```python
from build123d import *

# Parameters (mm, degrees)
F0_W     = 60
F0_H     = 100
F0_R     = 17.5
F1_DEPTH = 20
F2_W     = 100
F2_H     = 20
F2_R     = 5
F3_DEPTH = 100
F4_R     = 4.99999


# Not quite as in the source:
# - a fillet or chamfer is up to 0.001 mm smaller than in the source, because OpenCascade refuses the exact size


with BuildPart() as f1:
    # F0 (on Top) → F1 (new body)
    with BuildSketch(Plane.XY):
        Rectangle(F0_W, F0_H)
        Circle(F0_R, mode=Mode.SUBTRACT)
    extrude(amount=F1_DEPTH)

    # F2 (on face) → F3 (intersect)
    with BuildSketch(Plane.YZ.offset(30)):
        with Locations((0, 10)):
            Rectangle(F2_W, F2_H)
        with Locations((-35, 10)):
            Circle(F2_R, mode=Mode.SUBTRACT)
        with Locations((35, 10)):
            Circle(F2_R, mode=Mode.SUBTRACT)
    extrude(amount=-F3_DEPTH, mode=Mode.INTERSECT)

    # F4 (radius 5 in the source; OpenCascade refuses exactly that, so slightly less here)
    f4_edges = [f1.edges().sort_by_distance(p)[0] for p in [
        (30, 0, 20),
        (0, -50, 20),
        (-30, 0, 20),
        (0, 50, 20),
    ]]
    fillet(f4_edges, radius=F4_R)


solid = f1.part
```
For this review, take the finished solid that the model builds, in its own axes (mm). Round coordinates to 2 decimals unless told otherwise and drop trailing zeros. Write each loop counter-clockwise with the first axis right and the second up, starting at its lowest first coordinate (ties: lowest second). Pieces come first, ordered by that corner, then holes. Notation, with made-up numbers: (-15.75, 7.25) - (23.25, 7.25) arc R27 ccw to (23.25, 27.25) - close; hole circle Ø4 at (11.5, 39.25). An arc over 180 degrees is marked (long way). Write each question's results on one line, items separated by ' | '.
Item 1: For pin 1 (9 mm diameter, centred on y = 35, z = 10, fed in from +X), flat-tipped, find the tip position at first contact; note if it passes through.
Calculated:
pin 1: passes through
Item 2: Take a section at C-C on y = -31. State the section outline as (x, z) points, then the cut area to 3 significant figures.
Calculated:
outline: (-30, 0) - (30, 0) - (30, 7) - (-30, 7) - close; (-30, 13) - (30, 13) - (30, 15) arc R5 ccw to (25, 20) - (-25, 20) arc R5 ccw to (-30, 15) - close | area: 829 mm^2
Item 3: To check wall thickness, follow line 1 along Z through (x, y) = (7, 35); line 2 along Y through (x, z) = (27, 9.5); line 3 along Y through (x, z) = (0, 4.5). State the ranges of each line that lie inside material, in increasing order. Write a range as from..to.
Calculated:
line 1: z = 0..5, 15..20 | line 2: y = -50..-39.97, -30.03..30.03, 39.97..50 | line 3: y = -50..-17.5, 17.5..50
Item 4: Take a section at B-B on z = 10. State the section outline as (x, y) points.
Calculated:
outline: (-30, -50) - (30, -50) - (30, -40) - (-30, -40) - close; (-30, -30) - (30, -30) - (30, 30) - (-30, 30) - close; (-30, 40) - (30, 40) - (30, 50) - (-30, 50) - close; hole circle Ø35 at (0, 0)
Item 5: Take a section at D-D on x = -24. State the section outline as (y, z) points.
Calculated:
outline: (-50, 0) - (50, 0) - (50, 15) arc R5 ccw to (45, 20) - (-45, 20) arc R5 ccw to (-50, 15) - close; hole circle Ø10 at (-35, 10); hole circle Ø10 at (35, 10)
Item 6: Take a section at A-A on x = 0. State the section outline as (y, z) points, then the cut area to 3 significant figures.
Calculated:
outline: (-50, 0) - (-17.5, 0) - (-17.5, 20) - (-45, 20) arc R5 ccw to (-50, 15) - close; (17.5, 0) - (50, 0) - (50, 15) arc R5 ccw to (45, 20) - (17.5, 20) - close; hole circle Ø10 at (-35, 10); hole circle Ø10 at (35, 10) | area: 1,130 mm^2
Item 7: Draft analysis for pull direction Z (two halves, no side actions). For faces 1 (the face through (0, 50, 7)), 2 (the face through (0, 48, 19)), 3 (the face through (0, 30, 10)), state which applies: pulls with the +Z half, pulls with the -Z half, needs draft (parallel to the pull), parting line crosses it, or undercut.
Calculated:
face 1: needs draft | face 2: pulls with the +Z half | face 3: undercut
